Study the drawing (mm; zero at the part's minimum x, y, z) and answer. A direction names the side the tool comes from. Give positions to 0.01 mm unless a question says otherwise; leave off trailing zeros. Order: outer loops, then holes, each group sorted by start corner. A loop starts at its lowest first (then second) coordinate and runs counter-clockwise, first axis right, second up. Notation, with made-up numbers: (32.25, -35.5) - (82.25, -35.5) arc R20 ccw to (82.25, -9.5) - close; hole circle Ø4 at (75, -32). An arc over 180 degrees is marked (long way). Put each result on its own line as item: value.
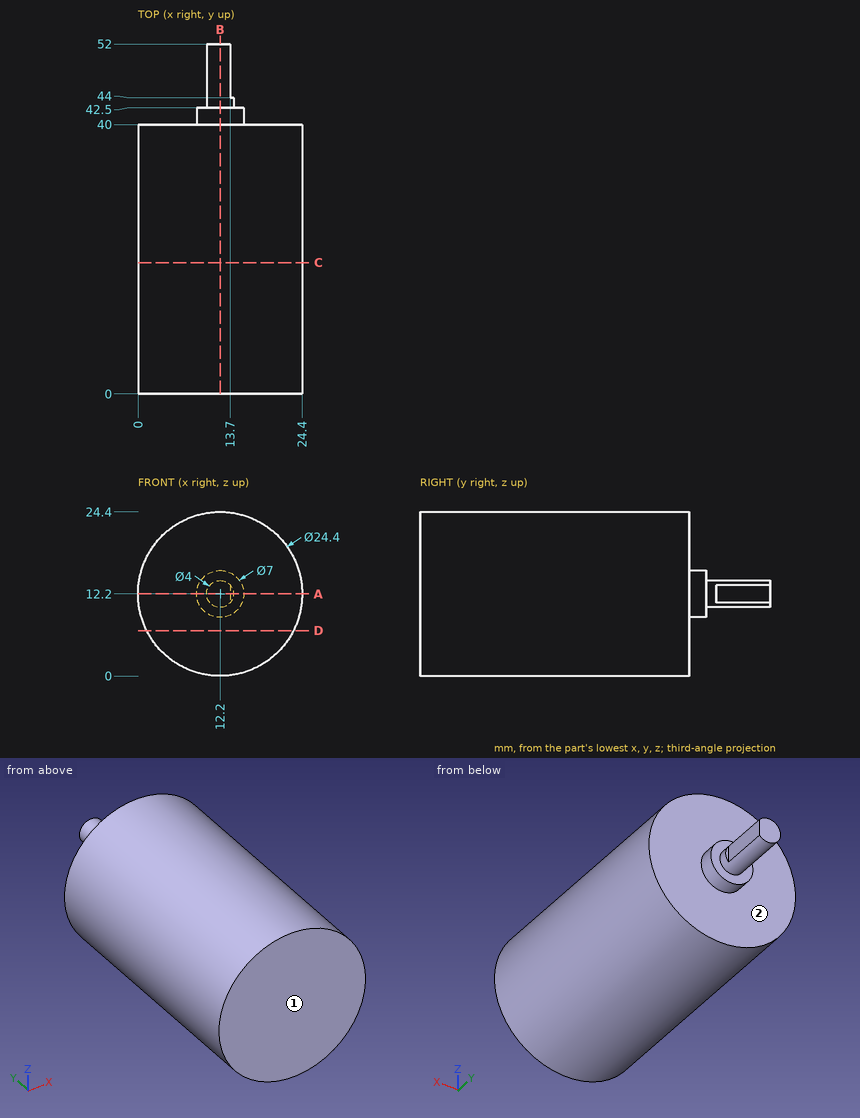
(1) Straight lines are drawn through the part: line 1 (Y direction, x = 17.5, z = 2.75); line 2 (X direction, y = 15, z = 17.5); line 3 (X direction, y = 23, z = 8.5). For each, find the intervals that lie inside material, in ascending order.
Geometry check:
line 1: y = 0 to 40
line 2: x = 1.21 to 23.19
line 3: x = 0.57 to 23.83
(2) A tool of negligible diameter and unlimited length cuts with its end or side. For the marked faces 1 and 2, from which of +Z, -Z, +X, -X, +Y, -Y can it reach the whole face along a straight path? Write none if from no direction.
Geometry check:
face 1: +Z, -Z, +X, -X, -Y
face 2: +Y
(3) Section A-A, the plane z = 12.2 is taken. Write down the section's boundary in (x, y).
Geometry check:
outline: (0, 0) - (24.4, 0) - (24.4, 40) - (15.7, 40) - (15.7, 42.5) - (14.2, 42.5) - (14.2, 44) - (13.7, 44) - (13.7, 52) - (10.2, 52) - (10.2, 42.5) - (8.7, 42.5) - (8.7, 40) - (0, 40) - close
(4) Section B-B, the plane x = 12.2 is taken. Write down the section's boundary in (y, z), then the cut area to 3 significant figures.
Geometry check:
outline: (0, 0) - (40, 0) - (40, 8.7) - (42.5, 8.7) - (42.5, 10.2) - (52, 10.2) - (52, 14.2) - (42.5, 14.2) - (42.5, 15.7) - (40, 15.7) - (40, 24.4) - (0, 24.4) - close
area: 1,030 mm²
(5) Section C-C, the plane y = 19.5 is taken. Write down the section's boundary in (x, z), then the cut area to 3 significant figures.
Geometry check:
outline: circle Ø24.4 at (12.2, 12.2)
area: 468 mm²
(6) Given pin 1 (1 mm diameter, centred on x = 15.5, y = 17.5, fed in from -Z); pin 2 (12 mm diameter, centred on x = 10.5, z = 17, fed in from +Y); pin 3 (4 mm diameter, centred on x = 20.5, z = 7.5, fed in from +Y); pin 4 (1.5 mm diameter, centred on x = 11.5, z = 9.5, fed in from +Y), each flat-ended and moving along its own axis, determine where each tip first touches the part or whether it passes through.
Geometry check:
pin 1: stops at z = 0.33
pin 2: stops at y = 52
pin 3: stops at y = 40
pin 4: stops at y = 42.5
(7) Section D-D, the plane z = 6.75 is taken. Write down the section's boundary in (x, y).
Geometry check:
outline: (1.28, 0) - (23.12, 0) - (23.12, 40) - (1.28, 40) - close
